For this review, take the finished solid that the model builds, in its own axes (mm). Give positions to 0.01 mm unless a question says otherwise; leave off trailing zeros. Write each loop counter-clockwise with the first axis right and the second up, starting at its lowest first coordinate (ties: lowest second). Pieces come first, ordered by that corner, then holes.
from build123d import *

# Parameters (mm, degrees)
SKETCH1_W           = 202
SKETCH1_H           = 202
BOSS_EXTRUDE1_DEPTH = 2
CUT_EXTRUDE1_REACH  = 144.85
SKETCH2_W           = 105
SKETCH2_H           = 105


with BuildPart() as part:
    # Sketch1 → Boss-Extrude1 (new body)
    with BuildSketch(Plane(origin=(0, 0, 0), x_dir=(1, 0, 0), z_dir=(0, 1, 0))):
        Rectangle(SKETCH1_W, SKETCH1_H)
    extrude(amount=BOSS_EXTRUDE1_DEPTH)

    # Sketch2 → Cut-Extrude1 (cut, up to next)
    with BuildSketch(Plane.XZ, mode=Mode.PRIVATE) as cut_extrude1_sk1:
        with Locations((-48.5, 0)):
            Rectangle(SKETCH2_W, SKETCH2_H)
    cut_extrude1_tool1 = extrude(cut_extrude1_sk1.sketch, amount=-CUT_EXTRUDE1_REACH, mode=Mode.PRIVATE) & part.part
    add(cut_extrude1_tool1.solids().sort_by_distance((-48.5, 0, 0))[0], mode=Mode.SUBTRACT)


solid = part.part
(1) For L1, parallel to Z at x = -22, y = 1.5; L2, parallel to X at y = 0.45, z = -8, list the stretches that pass through material, from the lowest coordinate up.
(2) Clearance check with a flat-ended pin moving along its axis: pin 1 Ø1 at (y, z) = (1, 6.5) entering from -X. State where the tip first meets the part, or that it passes through.
(3) We need section C-C (z = -22.5). Write out the cut boundary in (x, y), and give its area (3 significant figures).
(4) We need section A-A (x = -37). Write out the cut boundary in (y, z).
(5) We need section B-B (y = 0.6). Write out the cut boundary in (x, z), and give its area (3 significant figures).
The answers:
1. L1: z = -101 to -52.5, 52.5 to 101
1. L2: x = 4 to 101
2. pin 1: stops at x = 4
3. outline: (4, 0) - (101, 0) - (101, 2) - (4, 2) - close
3. area: 194 mm2
4. outline: (0, -101) - (2, -101) - (2, -52.5) - (0, -52.5) - close; (0, 52.5) - (2, 52.5) - (2, 101) - (0, 101) - close
5. outline: (-101, -101) - (101, -101) - (101, 101) - (-101, 101) - (-101, 52.5) - (4, 52.5) - (4, -52.5) - (-101, -52.5) - close
5. area: 29,800 mm2
